For this review, use the dimensioned drawing (mm, ordinates from the lowest corner) and the shaded views. A direction names the side the tool comes from. Give positions to 0.01 mm unless a question says otherwise; leave off trailing zeros. Write each loop counter-clockwise with the first axis right and the second up, starting at its lowest first coordinate (ties: lowest second). Pieces come first, ordered by that corner, then holes.
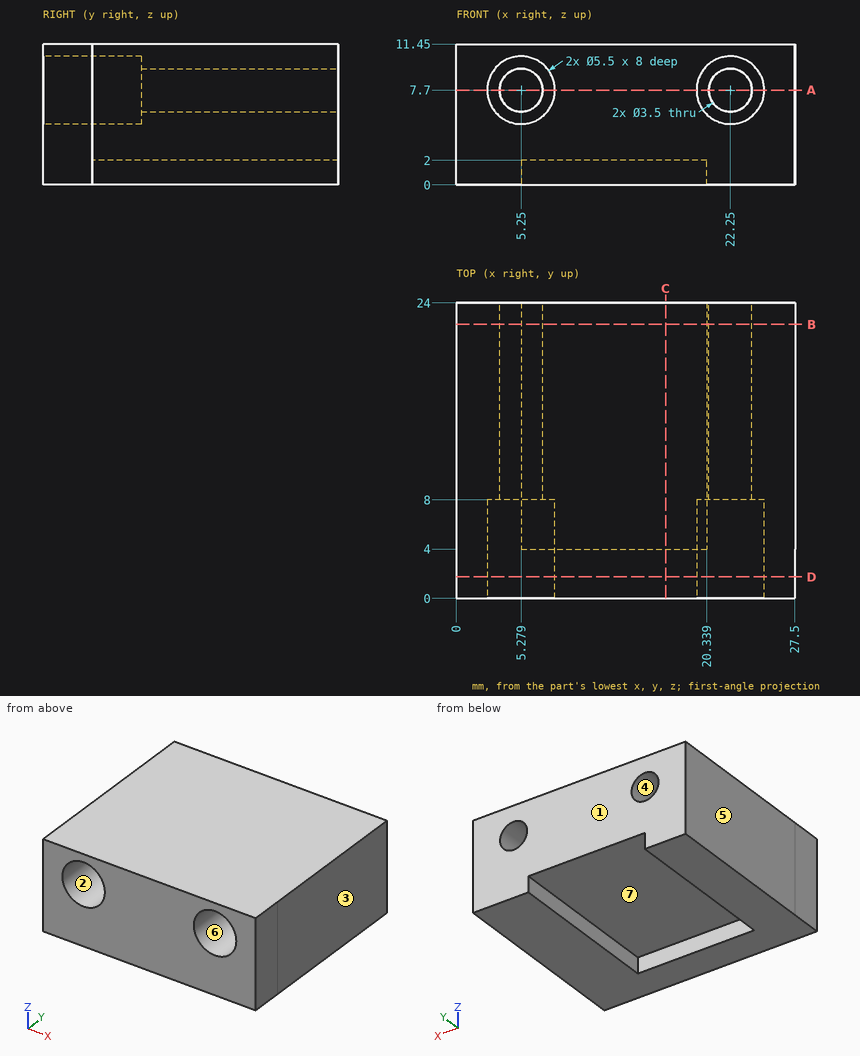
(1) Clearance check with a flat-ended pin moving along its axis: pin 1 Ø2 at (x, z) = (22.25, 7.7) entering from -Y. State where the tip first meets the part, or that it passes through.
(2) We need section A-A (z = 7.7). Write out the cut boundary in (x, y), and give its area (3 significant figures).
(3) We need section C-C (x = 17). Write out the cut boundary in (y, z).
(4) We need section D-D (y = 1.75). Write out the cut boundary in (x, z).
(5) For L1, parallel to X at y = 12.75, z = 9; L2, parallel to X at y = 10.25, z = 8.25; L3, parallel to Z at x = 12.5, y = 5.5, list the stretches that pass through material, from the lowest coordinate up.
(6) The part is to be moulded in two halves that separate along X. For the marked faces 1, 2, 3 and 4, say which applies: +X half, -X half, draft (parallel to the pull), parting line (faces both ways), or undercut.
(7) Tool access review of the marked faces 5, 6 and 7: name each direction out of +Z, -Z, +X, -X, +Y, -Y from which nothing blocks a thin tool from reaching the whole face with its end or side.
(8) We need section B-B (y = 22.25). Write out the cut boundary in (x, z).
The answers:
1. pin 1: passes through
2. outline: (0, 0) - (2.5, 0) - (2.5, 8) - (3.5, 8) - (3.5, 24) - (0, 24) - close; (7, 8) - (8, 8) - (8, 0) - (19.5, 0) - (19.5, 8) - (20.5, 8) - (20.5, 24) - (7, 24) - close; (24, 8) - (25, 8) - (25, 0) - (27.5, 0) - (27.5, 24) - (24, 24) - close
2. area: 460 mm2
3. outline: (0, 0) - (4, 0) - (4, 2) - (24, 2) - (24, 11.45) - (0, 11.45) - close
4. outline: (0, 0) - (27.5, 0) - (27.5, 11.45) - (0, 11.45) - close; hole circle Ø5.5 at (5.25, 7.7); hole circle Ø5.5 at (22.25, 7.7)
5. L1: x = 0 to 4.08, 6.42 to 21.08, 23.42 to 27.5
5. L2: x = 0 to 3.59, 6.91 to 20.59, 23.91 to 27.5
5. L3: z = 2 to 11.45
6. face 1: draft
6. face 2: undercut
6. face 3: +X half
6. face 4: undercut
7. face 5: +Z, -Z, -X, +Y, -Y
7. face 6: -Y
7. face 7: -Z, +Y
8. outline: (0, 0) - (5.28, 0) - (5.28, 2) - (20.34, 2) - (20.34, 0) - (27.5, 0) - (27.5, 11.45) - (0, 11.45) - close; hole circle Ø3.5 at (5.25, 7.7); hole circle Ø3.5 at (22.25, 7.7)
